from build123d import *

# Parameters (mm, degrees)
F0_W       = 11.7
F0_H       = 7.5
F0_W_2     = 8.7
F0_H_2     = 4.5
F1_DEPTH   = 12
F2_R       = 1
F3_SIZE2   = 2
F3_SIZE    = 0.75
F3_2_SIZE2 = 2
F3_2_SIZE  = 0.75
F4_R       = 10


with BuildPart() as f1:
    # F0 (on Top) → F1 (new body)
    with BuildSketch(Plane.XY):
        Rectangle(F0_W, F0_H)
        Rectangle(F0_W_2, F0_H_2, mode=Mode.SUBTRACT)
    extrude(amount=F1_DEPTH)

    # F2
    f2_edges = [f1.edges().sort_by_distance(p)[0] for p in [
        (5.85, -3.75, 6),
        (-5.85, -3.75, 6),
        (-5.85, 3.75, 6),
        (5.85, 3.75, 6),
    ]]
    fillet(f2_edges, radius=F2_R)

    # F3
    f3_edges = [f1.edges().sort_by_distance(p)[0] for p in [
        (0, -3.75, 12),
    ]]
    f3_side = f1.faces().sort_by_distance((0, -3.611025, 12))[0]
    chamfer(f3_edges, length=F3_SIZE, length2=F3_SIZE2, reference=f3_side)

    # F3#2
    f3_2_edges = [f1.edges().sort_by_distance(p)[0] for p in [
        (0, -3.75, 0),
    ]]
    f3_2_side = f1.faces().sort_by_distance((0, -3.611025, 0))[0]
    chamfer(f3_2_edges, length=F3_2_SIZE, length2=F3_2_SIZE2, reference=f3_2_side)

    # F4
    f4_edges = [f1.edges().sort_by_distance(p)[0] for p in [
        (0, -3.75, 2),
        (0, -3.75, 10),
    ]]
    fillet(f4_edges, radius=F4_R)


solid = f1.part
For this review, take the finished solid that the model builds, in its own axes (mm). A direction names the side the tool comes from. Give positions to 0.01 mm unless a question says otherwise; leave off trailing zeros. Loops run counter-clockwise (first coordinate to the right, second up) from the corner with the lowest first, then second, coordinate; pieces in that order, holes last. Notation, with made-up numbers: M 35,40 L 83,40 A36 ccw 83,75 Z; hole C -11,26 d7. An arc over 180 degrees is marked long. Put each result on its own line as item: value. Start each with the question number.
(1) The part is to be moulded in two halves that separate along Y. For faces 3 (the cylindrical face through (-5.565, 3.449, 6.031)), 4 (the flat face through (5.85, 0, 6)), 5 (the flat face through (0, -2.25, 6)), say which applies: +Y half, -Y half, draft (parallel to the pull), parting line (faces both ways), or undercut.
(2) Add section C-C, the plane z = 5.25. Write out the cut boundary in (x, y).
(3) Add section D-D, the plane y = 2.5. Write out the cut boundary in (x, z).
(4) Machinability: for faces 1 (the cylindrical face through (-0.068, 3.594, 2.054)), 2 (the flat face through (0, 2.25, 6)), which of the approach directions +Z, -Z, +X, -X, +Y, -Y give a long, thin tool a straight path to every point of the face, cutting with its end or side? Answer none if there is none.
(5) Add section B-B, the plane y = 0.5. Write out the cut boundary in (x, z).
(6) Add section A-A, the plane x = 1.5. Write out the cut boundary in (y, z).
(7) Wall thickness on L1, parallel to Y at x = -1.75, z = 5; L2, parallel to X at y = 1.5, z = 7.75: over which ranges is each line inside the solid? List them lowest first.
Result:
1. face 3: +Y half
1. face 4: draft
1. face 5: undercut
2. outline: M -5.85,-2.75 A1 ccw -4.85,-3.75 L 4.85,-3.75 A1 ccw 5.85,-2.75 L 5.85,2.75 A1 ccw 4.85,3.75 L -4.85,3.75 A1 ccw -5.85,2.75 Z; hole M -4.35,-2.25 L 4.35,-2.25 L 4.35,2.25 L -4.35,2.25 Z
3. outline: M -5.85,3.81 A10 ccw -5.21,0.3 L -5.1,0 L 5.1,0 L 5.21,0.3 A10 ccw 5.85,3.81 L 5.85,8.19 A10 ccw 5.21,11.7 L 5.1,12 L -5.1,12 L -5.21,11.7 A10 ccw -5.85,8.19 Z
4. face 1: -Z, +X, -X, +Y
4. face 2: +Z, -Z
5. outline: M -5.85,3.81 A10 ccw -5.21,0.3 L -5.1,0 L -4.35,0 L -4.35,12 L -5.1,12 L -5.21,11.7 A10 ccw -5.85,8.19 Z; M 4.35,0 L 5.1,0 L 5.21,0.3 A10 ccw 5.85,3.81 L 5.85,8.19 A10 ccw 5.21,11.7 L 5.1,12 L 4.35,12 Z
6. outline: M -3.75,3.81 A10 ccw -3.11,0.3 L -3,0 L -2.25,0 L -2.25,12 L -3,12 L -3.11,11.7 A10 ccw -3.75,8.19 Z; M 2.25,0 L 3,0 L 3.11,0.3 A10 ccw 3.75,3.81 L 3.75,8.19 A10 ccw 3.11,11.7 L 3,12 L 2.25,12 Z
7. L1: y = -3.75 to -2.25, 2.25 to 3.75
7. L2: x = -5.85 to -4.35, 4.35 to 5.85
